from build123d import *

# Parameters (mm, degrees)
F0_W           = 76.2
F0_H           = 150
F1_DEPTH       = 19.05
F3_D           = 3.4
F3_CBORE_D     = 6.5
F3_CBORE_DEPTH = 3
F5_D           = 2.5
F5_DEPTH       = 20.55
F5_TIP         = 0.7510757738


with BuildPart() as f1:
    # F0 (on Front) → F1 (new body)
    with BuildSketch(Plane.XZ):
        with Locations((38.1, 75)):
            Rectangle(F0_W, F0_H)
    extrude(amount=F1_DEPTH)

    # F3 (through all)
    with Locations(Plane.XZ.offset(19.05)):
        with Locations((15.875, 117.275), (15.875, 92.275), (15.875, 28.375), (15.875, 3.375), (60.325, 3.375), (60.325, 28.375), (60.325, 92.275), (60.325, 117.275)):
            CounterBoreHole(F3_D / 2, F3_CBORE_D / 2, F3_CBORE_DEPTH)

    # F5
    with Locations(Plane.XZ.offset(19.05)):
        with Locations((7.9375, 135), (7.9375, 95), (7.9375, 55), (7.9375, 15), (68.2625, 15), (68.2625, 55), (68.2625, 95), (68.2625, 135)):
            Hole(F5_D / 2, depth=F5_DEPTH)
            with Locations((0, 0, -(F5_DEPTH + F5_TIP / 2))):  # 118° drill point
                Cone(0, F5_D / 2, F5_TIP, mode=Mode.SUBTRACT)


solid = f1.part
Part model, mm, in its own coordinate system. A direction names the side the tool comes from. Coordinates: 2 decimals unless noted, no trailing zeros. Use a Markdown table: item, result. Add a question column.
Q1. Which spindle directions (+Z, -Z, +X, -X, +Y, -Y) get a long thin tool onto all of the face, cutting with end or side? Do faces 1 (the cylindrical face through (61.6, -7.9, 118.4)), 2 (the flat face through (62, -16.05, 27)). Say none if no direction does.
Q2. Probe L1, parallel to X at y = -6.5, z = 135; L2, parallel to X at y = -13.5, z = 118; L3, parallel to Z at x = 9, y = -11. List the from-to ranges inside material, lowest first.
Q3. Pin check, flat tips, straight feed: P1, Ø7, axis at x = 17, z = 90.5, coming from the -Y side; P2, Ø2, axis at x = 14.5, z = 118.5, coming from the -Y side; P3, Ø2, axis at x = 68.26, z = 95, coming from the +Y side. Stop position of each tip, or through.
Q4. Mould opens along Z. For faces 3 (the flat face through (17.3, -16.05, 115.9)), 4 (the flat face through (76.2, -9, 74)), 5 (the flat face through (38, -9, 0)), 6 (the cylindrical face through (59.902, -17.571, 120.497)) say: +Z half, -Z half, draft (parallel to the pull), parting line (faces both ways), or undercut.
Worked out:
| question | item | result |
|---|---|---|
| 1 | face 1 | +Y, -Y |
| 1 | face 2 | -Y |
| 2 | L1 | x = 0 to 6.69, 9.19 to 67.01, 69.51 to 76.2 |
| 2 | L2 | x = 0 to 14.34, 17.41 to 58.79, 61.86 to 76.2 |
| 2 | L3 | z = 0 to 14.34, 15.66 to 54.34, 55.66 to 94.34, 95.66 to 134.34, 135.66 to 150 |
| 3 | P1 | stops at y = -19.05 |
| 3 | P2 | stops at y = -16.05 |
| 3 | P3 | passes through |
| 4 | face 3 | undercut |
| 4 | face 4 | draft |
| 4 | face 5 | -Z half |
| 4 | face 6 | undercut |
